Source: three-view drawing plus pictorial views. Frame: mm from the lowest corner of the part. A direction names the side the tool comes from. Coordinates: 2 decimals unless noted, no trailing zeros. Write each loop counter-clockwise with the first axis right and the second up, starting at its lowest first coordinate (ties: lowest second). Pieces come first, ordered by that corner, then holes. Notation, with made-up numbers: M 7,-30.5 L 14,-30.5 A21 cw 14,7.5 Z; hole C 79,-34.75 d6. An arc over 180 degrees is marked long. Write item = value, one per line. Start each with the question number.
Item 1: First-contact query: pin 1 Ø5 at (x, z) = (26, 44.5) entering from -Y; pin 2 Ø1 at (y, z) = (32.5, 29) entering from -X; pin 3 Ø8 at (x, z) = (42.5, 57.5) entering from +Y. Flat tips, straight axial feed; report the tip coordinate or a pass-through.
Item 2: Section B-B on x = 73. Output: boundary loops of the cut face in (y, z).
Item 3: Section C-C on z = 45. Output: boundary loops of the cut face in (x, y), plus the area to 3 significant figures.
Item 4: Pull-direction query (Z, two-part tool) for the marked faces 3, 4, 5 and 6; classes: +Z half, -Z half, draft (parallel to the pull), parting line (faces both ways), or undercut.
Item 5: Section D-D on y = 27. Output: boundary loops of the cut face in (x, z), plus the area to 3 significant figures.
Item 6: Section A-A on y = 145. Output: boundary loops of the cut face in (x, z), plus the area to 3 significant figures.
Item 7: Reachability of the marked faces 1 and 2 from +Z, -Z, +X, -X, +Y, -Y: full face, straight path, thin tool, end or side. Return the list, or none.
Item 8: Ray query, L1, parallel to Z at x = 75.5, y = 145; L2, parallel to Y at x = 62, z = 44; L3, parallel to X at y = 75, z = 12. Return the intervals inside material, ascending. Write a range as [from, to].
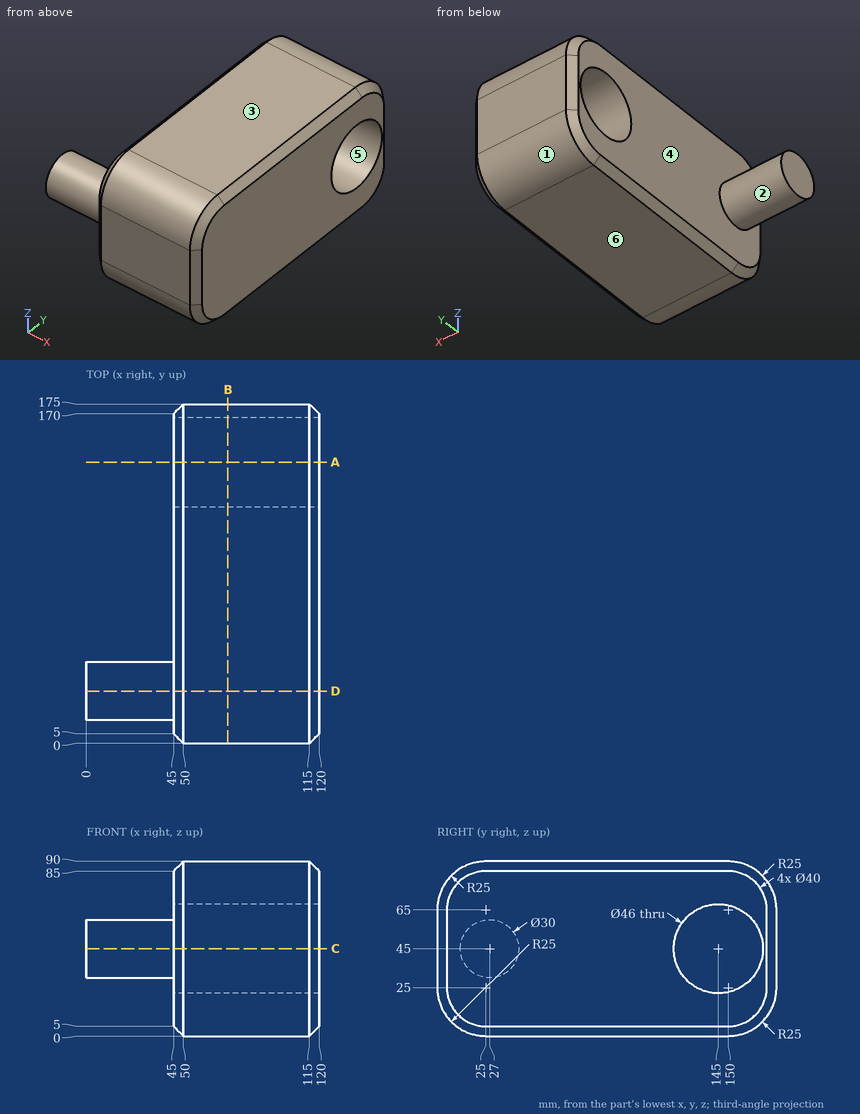
Responses:
q1.pin_1 = 12
q1.pin_2 = 45
q1.pin_3 = 171.5
q2.outline = M 0,25 A25 ccw 25,0 L 150,0 A25 ccw 175,25 L 175,65 A25 ccw 150,90 L 25,90 A25 ccw 0,65 Z; hole C 145,45 d46
q3.outline = M 0,12 L 45,12 L 45,5 L 50,0 L 115,0 L 120,5 L 120,122 L 45,122 L 45,42 L 0,42 Z; M 45,168 L 120,168 L 120,170 L 115,175 L 50,175 L 45,170 Z
q3.area = 11,000 mm²
q4.face_3 = +Z half
q4.face_4 = draft
q4.face_5 = undercut
q4.face_6 = -Z half
q5.outline = M 0,30 L 45,30 L 45,5 L 50,0 L 115,0 L 120,5 L 120,85 L 115,90 L 50,90 L 45,85 L 45,60 L 0,60 Z
q5.area = 8,050 mm²
q6.outline = M 45,5 L 50,0 L 115,0 L 120,5 L 120,22 L 45,22 Z; M 45,68 L 120,68 L 120,85 L 115,90 L 50,90 L 45,85 Z
q6.area = 3,250 mm²
q7.face_1 = -Z, +X, -X, +Y
q7.face_2 = -X
q8.L1 = [0, 22], [68, 90]
q8.L2 = [0, 122.02], [167.98, 175]
q8.L3 = [45, 120]
